```python
from build123d import *

# Parameters (mm, degrees)
F0_W     = 15.875
F0_H     = 15.875
F1_DEPTH = 38.1
F2_R     = 4.1275
F3_DEPTH = 4.826
F4_SIZE  = 1.778
F5_T     = -1.5875
F6_R     = 0.508


with BuildPart() as f1:
    # F0 (on Front) → F1 (new body)
    with BuildSketch(Plane.XZ):
        Rectangle(F0_W, F0_H)
    extrude(amount=F1_DEPTH)

    # F2 (on face) → F3 (join)
    with BuildSketch(Plane.XZ.offset(38.1)):
        Circle(F2_R)
    extrude(amount=F3_DEPTH)

    # F4
    f4_edges = [f1.edges().sort_by_distance(p)[0] for p in [
        (-4.1275, -42.926, 0),
    ]]
    chamfer(f4_edges, length=F4_SIZE)

    # F5
    f5_openings = [f1.faces().sort_by_distance(p)[0] for p in [
        (0, 0, 0),
    ]]
    offset(amount=F5_T, openings=f5_openings, kind=Kind.INTERSECTION)

    # F6
    f6_edges = [f1.edges().sort_by_distance(p)[0] for p in [
        (0, -38.1, 7.9375),
        (-7.9375, -38.1, 0),
        (0, -38.1, -7.9375),
        (7.9375, -38.1, 0),
        (-7.9375, -19.05, 7.9375),
        (-7.9375, -19.05, -7.9375),
        (7.9375, -19.05, 7.9375),
        (7.9375, -19.05, -7.9375),
        (0, 0, -7.9375),
        (7.9375, 0, 0),
        (0, 0, 7.9375),
        (-7.9375, 0, 0),
    ]]
    fillet(f6_edges, radius=F6_R)


solid = f1.part
```
Work out the finished part from the listing and answer in its coordinate system (mm). A direction names the side the tool comes from. Round coordinates to 2 decimals unless told otherwise and drop trailing zeros. Loops run counter-clockwise (first coordinate to the right, second up) from the corner with the lowest first, then second, coordinate; pieces in that order, holes last. Notation, with made-up numbers: M -11.5,11.5 L 12.5,11.5 A14 ccw 12.5,37.5 Z; hole C 8.25,37 d7. An arc over 180 degrees is marked long. One line per question, with ' | ' between items.
Q1. A tool of negligible diameter and unlimited length cuts with its end or side. For faces 4 (the flat face through (3.2, -38.1, 3.4)), 5 (the flat face through (-7.938, -19, 0)), 6 (the flat face through (0, -18, -6.35)), from which of +Z, -Z, +X, -X, +Y, -Y can it reach the whole face along a straight path? Write none if from no direction.
Conclusion:
face 4: -Y | face 5: +Z, -Z, -X, +Y, -Y | face 6: +Y
Q2. Find section C-C, the plane z = 0. Give the vertices of the cut face in (x, y).
Conclusion:
outline: M -7.94,-37.59 A0.51 ccw -7.43,-38.1 L -4.13,-38.1 L -4.13,-41.15 L -2.35,-42.93 L 2.35,-42.93 L 4.13,-41.15 L 4.13,-38.1 L 7.43,-38.1 A0.51 ccw 7.94,-37.59 L 7.94,-0.51 A0.51 ccw 7.43,0 L 6.35,0 L 6.35,-36.51 L 2.54,-36.51 L 2.54,-40.49 L 1.69,-41.34 L -1.69,-41.34 L -2.54,-40.49 L -2.54,-36.51 L -6.35,-36.51 L -6.35,0 L -7.43,0 A0.51 ccw -7.94,-0.51 Z
Q3. Find section D-D, the plane x = 0. Give the vertices of the cut face in (y, z), then the cut area to 3 significant figures.
Conclusion:
outline: M -42.93,-2.35 L -41.15,-4.13 L -38.1,-4.13 L -38.1,-7.43 A0.51 ccw -37.59,-7.94 L -0.51,-7.94 A0.51 ccw 0,-7.43 L 0,-6.35 L -36.51,-6.35 L -36.51,-2.54 L -40.49,-2.54 L -41.34,-1.69 L -41.34,1.69 L -40.49,2.54 L -36.51,2.54 L -36.51,6.35 L 0,6.35 L 0,7.43 A0.51 ccw -0.51,7.94 L -37.59,7.94 A0.51 ccw -38.1,7.43 L -38.1,4.13 L -41.15,4.13 L -42.93,2.35 Z | area: 154 mm2
Q4. The mould has two halves that part along Z. Classify faces 1 (the flat face through (0, -19, -7.938)), 2 (the flat face through (-7, 0, 0)), 3 (the flat face through (-6.35, -18, 0)): +Z half, -Z half, draft (parallel to the pull), parting line (faces both ways), or undercut.
Conclusion:
face 1: -Z half | face 2: draft | face 3: undercut
Q5. Find section A-A, the plane x = -6.75. Give the vertices of the cut face in (y, z).
Conclusion:
outline: M -38.1,-7.43 A0.51 ccw -37.59,-7.94 L -0.51,-7.94 A0.51 ccw 0,-7.43 L 0,7.43 A0.51 ccw -0.51,7.94 L -37.59,7.94 A0.51 ccw -38.1,7.43 Z
Q6. Find section B-B, the plane y = -8. Give the vertices of the cut face in (x, z), then the cut area to 3 significant figures.
Conclusion:
outline: M -7.94,-7.43 A0.51 ccw -7.43,-7.94 L 7.43,-7.94 A0.51 ccw 7.94,-7.43 L 7.94,7.43 A0.51 ccw 7.43,7.94 L -7.43,7.94 A0.51 ccw -7.94,7.43 Z; hole M -6.35,-6.35 L 6.35,-6.35 L 6.35,6.35 L -6.35,6.35 Z | area: 90.5 mm2
Q7. Each of these flat-tipped pins is pushed along its axis until it touches: pin 1 Ø2.5 at (x, z) = (0, 0) entering from +Y; pin 2 Ø4 at (x, z) = (4, -2) entering from -Y; pin 3 Ø2 at (x, z) = (1.5, 3.5) entering from +Y. Where does it stop, or does it pass through?
Conclusion:
pin 1: stops at y = -41.34 | pin 2: stops at y = -42.8 | pin 3: stops at y = -36.51
Q8. Consider line 1 along Z through (x, y) = (3, -29); line 2 along Z through (x, y) = (0, -38.7). Determine where each line is inside the solid, lowest interval first. Write a range as from..to.
Conclusion:
line 1: z = -7.94..-6.35, 6.35..7.94 | line 2: z = -4.13..-2.54, 2.54..4.13
